```python
from build123d import *

# Parameters (mm, degrees)
BOSS_EXTRUDE1_DEPTH     = 60
CUT_EXTRUDE1_DEPTH      = 9
CUT_EXTRUDE1_DEPTH_BACK = 1
CUT_EXTRUDE2_DEPTH      = 61.307545133
CUT_EXTRUDE2_DEPTH_BACK = 61.307545133
SKETCH3_R               = 1


with BuildPart() as part:
    # Sketch1 → Boss-Extrude1 (new body)
    with BuildSketch(Plane.XY):
        with BuildLine():
            ThreePointArc((5.744562647, 4), (0, 7), (-5.744562647, 4))
            Line((-5.744562647, 4), (5.744562647, 4))
        make_face()
    extrude(amount=BOSS_EXTRUDE1_DEPTH)

    # Sketch2 → Cut-Extrude1 (cut, two sides: drawn at the far end of the back side and taken through both)
    with BuildSketch(Plane.XZ.offset(-4).offset(-CUT_EXTRUDE1_DEPTH_BACK)):
        Polygon((-2.502029768, 57), (-1.34732923, 55), (0.962071847, 55), (2.116772385, 57), (0.962071847, 59), (-1.34732923, 59), align=None)
        Polygon((-2.502029768, 3), (-1.34732923, 1), (0.962071847, 1), (2.116772385, 3), (0.962071847, 5), (-1.34732923, 5), align=None)
    extrude(amount=CUT_EXTRUDE1_DEPTH + CUT_EXTRUDE1_DEPTH_BACK, mode=Mode.SUBTRACT)

    # Sketch3 → Cut-Extrude2 (cut, two sides: drawn at the far end of the back side and taken through both)
    with BuildSketch(Plane.XZ.offset(-5).offset(-CUT_EXTRUDE2_DEPTH_BACK)):
        with Locations(Location((0, 2.888785773, 0), (0, 0, 270))):
            Circle(SKETCH3_R)
        with Locations(Location((0, 56.888785773, 0), (0, 0, 270))):
            Circle(SKETCH3_R)
    extrude(amount=CUT_EXTRUDE2_DEPTH + CUT_EXTRUDE2_DEPTH_BACK, mode=Mode.SUBTRACT)


solid = part.part
```
Can you work these out from the model? Positions are in its coordinate system, mm. A direction names the side the tool comes from. Round coordinates to 2 decimals unless told otherwise and drop trailing zeros. Loops run counter-clockwise (first coordinate to the right, second up) from the corner with the lowest first, then second, coordinate; pieces in that order, holes last.
Item 1: Suppose I cut it at D-D, the plane x = 3. Write out the boundary of the cut face in (y, z).
Item 2: Suppose I cut it at A-A, the plane x = 0. Write out the boundary of the cut face in (y, z).
Item 3: Please list where these lines run through material, in increasing order: L1, parallel to Z at x = 0, y = 5.5; L2, parallel to Y at x = 4, z = 56; L3, parallel to Z at x = -1.5, y = 4.5.
Item 4: Will these pins go through, and if not, where does the flat tip stop? pin 1 Ø0.5 at (x, y) = (0, 4.5) entering from -Z; pin 2 Ø1 at (y, z) = (6.5, 29) entering from +X; pin 3 Ø1.2 at (x, z) = (0, 56.89) entering from +Y; pin 4 Ø1.5 at (x, z) = (-2.5, 41) entering from +Y.
Item 5: Suppose I cut it at B-B, the plane z = 12. Write out the boundary of the cut face in (x, y).
Item 6: Suppose I cut it at C-C, the plane y = 6.3. Write out the boundary of the cut face in (x, z).
Item 7: Which directions (+Z, -Z, +X, -X, +Y, -Y) give clear straight access to the entire face, cutting with the end or side of a thin tool? Please do faces 1 (the cylindrical face through (0.3, 6.014, 55.935)), 2 (the flat face through (1.531, 4.507, 1.986)).
Item 8: If we mould it in two halves opening along X, with no side actions, what happens to faces 3 (the flat face through (0, 5, 0)), 4 (the flat face through (-1, 5, 4)), 5 (the cylindrical face through (0, 7, 30))? For each: +X half, -X half, draft (parallel to the pull), parting line (faces both ways), or undercut.
Reported:
1. outline: (4, 0) - (6.32, 0) - (6.32, 60) - (4, 60) - close
2. outline: (4, 0) - (7, 0) - (7, 1.89) - (5, 1.89) - (5, 1) - (4, 1) - close; (4, 5) - (5, 5) - (5, 3.89) - (7, 3.89) - (7, 55.89) - (5, 55.89) - (5, 55) - (4, 55) - close; (4, 59) - (5, 59) - (5, 57.89) - (7, 57.89) - (7, 60) - (4, 60) - close
3. L1: z = 0 to 1.89, 3.89 to 55.89, 57.89 to 60
3. L2: y = 4 to 5.74
3. L3: z = 0 to 1.26, 4.74 to 55.26, 58.74 to 60
4. pin 1: stops at z = 0
4. pin 2: stops at x = 3.61
4. pin 3: passes through
4. pin 4: stops at y = 6.78
5. outline: (-5.74, 4) - (5.74, 4) arc R7 ccw to start
6. outline: (-3.05, 0) - (3.05, 0) - (3.05, 60) - (-3.05, 60) - close; hole circle Ø2 at (0, 2.89); hole circle Ø2 at (0, 56.89)
7. face 1: +Y, -Y
7. face 2: -Y
8. face 3: draft
8. face 4: undercut
8. face 5: parting line
